Part model, mm, in its own coordinate system. A direction names the side the tool comes from. Coordinates: 2 decimals unless noted, no trailing zeros. Loops run counter-clockwise (first coordinate to the right, second up) from the corner with the lowest first, then second, coordinate; pieces in that order, holes last. Notation, with made-up numbers: (3, 62) -> (15, 62) arc R21 ccw to (15, 87) -> close; hole circle Ø9 at (-28.75, -16.75). An arc over 180 degrees is marked (long way). One line per item, written item: value. Start each with the question number.
from build123d import *

# Parameters (mm, degrees)
F1_DEPTH = 3


with BuildPart() as f1:
    # F0 (on Front) → F1 (new body)
    with BuildSketch(Plane.XZ):
        with BuildLine():
            Line((245, 30), (-245, 30))
            Line((-245, 30), (-245, 0))
            ThreePointArc((-245, 0), (-224.293242, -28.524299), (-190.757623, -17.672214))
            ThreePointArc((-190.757623, -17.672214), (-177.603175, -8.412973), (-161.530789, -9.084856))
            Line((-161.530789, -9.084856), (-116.524853, -26.506509))
            ThreePointArc((-116.524853, -26.506509), (-107.5, -28.192306), (-98.475147, -26.506509))
            Line((-98.475147, -26.506509), (-53.469211, -9.084856))
            ThreePointArc((-53.469211, -9.084856), (-37.396825, -8.412973), (-24.242377, -17.672214))
            ThreePointArc((-24.242377, -17.672214), (0, -30), (24.242377, -17.672214))
            ThreePointArc((24.242377, -17.672214), (37.396825, -8.412973), (53.469211, -9.084856))
            Line((53.469211, -9.084856), (98.475147, -26.506509))
            ThreePointArc((98.475147, -26.506509), (107.5, -28.192306), (116.524853, -26.506509))
            Line((116.524853, -26.506509), (161.530789, -9.084856))
            ThreePointArc((161.530789, -9.084856), (177.603175, -8.412973), (190.757623, -17.672214))
            ThreePointArc((190.757623, -17.672214), (224.293242, -28.524299), (245, 0))
            Line((245, 0), (245, 30))
        make_face()
    extrude(amount=F1_DEPTH)


solid = f1.part
1) Tool access for faces 3 (the flat face through (-3, 0, 7)), 4 (the flat face through (-76.29, -1.48, -17.92)): list every direction of +Z, -Z, +X, -X, +Y, -Y with a clear straight run to the whole face (end or side of a thin tool).
2) Pin check, flat tip, straight feed: pin 1 Ø12 at (x, z) = (116, -11.5) entering from +Y. Stop position of the tip, or through.
3) Slice it at B-B (x = -76). Give the cut face in (y, z), then the cut area to 3 significant figures.
4) Slice it at A-A (y = -1.85). Give the cut face in (x, z), then the cut area to 3 significant figures.
5) Slice it at C-C (x = 90). Give the cut face in (y, z).
6) Pull direction X, two halves, no side cores. Call faces 1 (the flat face through (-3, -3, 7)), 2 (the flat face through (138.71, -1.48, -17.92)): +X half, -X half, draft (parallel to the pull), parting line (faces both ways), or undercut.
7) Probe line 1 (Z direction, x = -225, y = -1.7); line 2 (Z direction, x = -172, y = -0.7); line 3 (X direction, y = -0.2, z = -4.5). List the from-to ranges inside material, lowest first. Write a range as from..to.
Check sheet entries:
1. face 3: +Z, -Z, +X, -X, +Y
1. face 4: -Z, +Y, -Y
2. pin 1: stops at y = 0
3. outline: (-3, -17.81) -> (0, -17.81) -> (0, 30) -> (-3, 30) -> close
3. area: 143 mm^2
4. outline: (-245, 0) arc R30 ccw to (-190.76, -17.67) arc R25 cw to (-161.53, -9.08) -> (-116.52, -26.51) arc R25 ccw to (-98.48, -26.51) -> (-53.47, -9.08) arc R25 cw to (-24.24, -17.67) arc R30 ccw to (24.24, -17.67) arc R25 cw to (53.47, -9.08) -> (98.48, -26.51) arc R25 ccw to (116.52, -26.51) -> (161.53, -9.08) arc R25 cw to (190.76, -17.67) arc R30 ccw to (245, 0) -> (245, 30) -> (-245, 30) -> close
4. area: 24,000 mm^2
5. outline: (-3, -23.23) -> (0, -23.23) -> (0, 30) -> (-3, 30) -> close
6. face 1: draft
6. face 2: undercut
7. line 1: z = -28.28..30
7. line 2: z = -7.44..30
7. line 3: x = -244.66..244.66
